Design review of the part built by this model. Coordinates are the model's own, in mm. A direction names the side the tool comes from. Coordinates: 2 decimals unless noted, no trailing zeros. Order: outer loops, then holes, each group sorted by start corner. A loop starts at its lowest first (then second) coordinate and runs counter-clockwise, first axis right, second up. Notation, with made-up numbers: M -1.5,39 L 30.5,39 A12 ccw 30.5,52 Z; hole C 14.5,86.5 d8. An arc over 180 degrees is marked long. Answer as a JSON object with one key per item and string values.
from build123d import *

# Parameters (mm, degrees)
SALIENTE_EXTRUIR1_DEPTH = 30
CORTAR_EXTRUIR1_DEPTH   = 30


with BuildPart() as part:
    # Croquis1 → Saliente-Extruir1 (new body)
    with BuildSketch(Plane.XY):
        with BuildLine():
            Line((0, 0), (20, 0))
            Line((20, 0), (20, -90))
            Line((20, -90), (32.5, -90))
            ThreePointArc((32.5, -90), (62.5, -120), (32.5, -150))
            Line((32.5, -150), (-12.5, -150))
            ThreePointArc((-12.5, -150), (-42.5, -120), (-12.5, -90))
            Line((-12.5, -90), (0, -90))
            Line((0, -90), (0, 0))
        make_face()
        with BuildLine():
            Line((32.5, -140), (-12.5, -140))
            ThreePointArc((-12.5, -140), (-32.5, -120), (-12.5, -100))
            Line((-12.5, -100), (32.5, -100))
            Line((32.5, -100), (32.5, -140))
        make_face(mode=Mode.SUBTRACT)
    extrude(amount=SALIENTE_EXTRUIR1_DEPTH)

    # Croquis3 → Cortar-Extruir1 (cut)
    with BuildSketch(Plane(origin=(20, 0, 0), x_dir=(0, 0, -1), z_dir=(1, 0, 0))):
        with BuildLine():
            Line((-10.497811767, -10), (-10.497811767, -80))
            ThreePointArc((-10.497811767, -80), (-15.497811767, -85), (-20.497811767, -80))
            Line((-20.497811767, -80), (-20.497811767, -10))
            ThreePointArc((-20.497811767, -10), (-15.497811767, -5), (-10.497811767, -10))
        make_face()
    extrude(amount=-CORTAR_EXTRUIR1_DEPTH, mode=Mode.SUBTRACT)


solid = part.part
1) Add section B-B (x = 9.5). State the section outline as (y, z) points, and give its area (3 significant figures).
Taken from the geometry:
{"outline": "M -150,0 L -140,0 L -140,30 L -150,30 Z; M -100,0 L 0,0 L 0,30 L -100,30 Z; hole M -80,10.5 L -10,10.5 A5 ccw -10,20.5 L -80,20.5 A5 ccw Z", "area": "2,520 mm2"}
2) Add section D-D (z = 3.25). State the section outline as (x, y) points.
Taken from the geometry:
{"outline": "M -12.5,-150 L 32.5,-150 A30 ccw 32.5,-90 L 20,-90 L 20,0 L 0,0 L 0,-90 L -12.5,-90 A30 ccw Z; hole M -12.5,-140 L 32.5,-140 L 32.5,-100 L -12.5,-100 A20 ccw Z"}
3) Insertion check: pin 1 Ø1.5 at (y, z) = (-70.5, 23) entering from +X; pin 2 Ø1 at (y, z) = (-129, 10.5) entering from +X; pin 3 Ø3 at (y, z) = (-18.5, 18.5) entering from +X; pin 4 Ø15 at (y, z) = (-61.5, 21.5) entering from -X. Each pin has a flat end and moves straight along its axis. Give the tip position at first contact, or say it passes through.
Taken from the geometry:
{"pin 1": "stops at x = 20", "pin 2": "stops at x = 61.27", "pin 3": "passes through", "pin 4": "stops at x = 0"}
4) Tool access review of faces 1 (the cylindrical face through (10.1, -85, 15.4)), 2 (the flat face through (10, -100, 15)), 3 (the flat face through (-6, -90, 15)): name each direction out of +Z, -Z, +X, -X, +Y, -Y from which nothing blocks a thin tool from reaching the whole face with its end or side.
Taken from the geometry:
{"face 1": "+X, -X", "face 2": "+Z, -Z", "face 3": "+Z, -Z, -X, +Y"}
5) Add section C-C (y = -120). State the section outline as (x, z) points, and give its area (3 significant figures).
Taken from the geometry:
{"outline": "M -42.5,0 L -32.5,0 L -32.5,30 L -42.5,30 Z; M 32.5,0 L 62.5,0 L 62.5,30 L 32.5,30 Z", "area": "1,200 mm2"}
6) Mouldability with a two-part tool opening along Y and no side actions: class faces 4 (the flat face through (14, -91, 0)), 5 (the cylindrical face through (-32.495, -120.44, 14.79)), 6 (the flat face through (26, -90, 15)), 7 (the flat face through (10, -140, 15)) as released by +Y, released by -Y, zero draft, split by the parting line, or undercut.
Taken from the geometry:
{"face 4": "zero draft", "face 5": "undercut", "face 6": "released by +Y", "face 7": "undercut"}
7) To check wall thickness, follow L1, parallel to Y at x = 1.5, z = 23; L2, parallel to Z at x = 8, y = -30.5; L3, parallel to Y at x = -8, z = 8.25. State the ranges of each line that lie inside material, in increasing order.
Taken from the geometry:
{"L1": "y = -150 to -140, -100 to 0", "L2": "z = 0 to 10.5, 20.5 to 30", "L3": "y = -150 to -140, -100 to -90"}
8) Add section A-A (x = -5.5). State the section outline as (y, z) points, and give its area (3 significant figures).
Taken from the geometry:
{"outline": "M -150,0 L -140,0 L -140,30 L -150,30 Z; M -100,0 L -90,0 L -90,30 L -100,30 Z", "area": "600 mm2"}
